Here's how the part is built. I have some questions about the finished solid (model axes, mm). Face numbers are marked on the shaded views. Coordinates: 2 decimals unless noted, no trailing zeros. Loops run counter-clockwise (first coordinate to the right, second up) from the corner with the lowest first, then second, coordinate; pieces in that order, holes last. Notation, with made-up numbers: (14, 0) -> (53, 0) arc R28 ccw to (53, 39) -> close; hole circle Ø8 at (43.25, 59). An arc over 180 degrees is marked (long way). Answer as a JSON object with one key per item and string values. Group by question number.
1) I'm going to push flat-ended pins straight in: pin 1 (5 mm diameter, centred on x = -3, z = 4, fed in from +Y); pin 2 (3 mm diameter, centred on x = -8.5, z = -15.5, fed in from -Y); pin 3 (3 mm diameter, centred on x = -3, y = 12, fed in from +Z). Where does each tip first touch, or does it pass through?
2) I want a section at C-C (y = 32.5). Write out the boundary of the cut face in (x, z) (3 decimals).
3) I want a section at B-B (z = 0). Count the separate pieces of the cut face and the enclosed holes in it, then the cut area to 3 significant figures.
4) I need wall thicknesses on probe 1 along Y at (x, z) = (-15.25, 0) (3 decimals); probe 2 along X at (y, z) = (12, 33); probe 3 along Y at (x, z) = (-4.75, 0). Which ranges of each line are inside material? Lowest first, please. Write a range as [from, to].
5) If we mould it in two halves opening along X, with no side actions, what happens to the marked faces 1, 2 and 3? For each: +X half, -X half, draft (parallel to the pull), parting line (faces both ways), or undercut.
6) I want a section at A-A (x = -2.5). Write out the boundary of the cut face in (y, z), then the cut area to 3 significant figures.
```python
from build123d import *

# Parameters (mm, degrees)
M2_5X0_45_TAPPED_HOLE2_D     = 2.05
M2_5X0_45_TAPPED_HOLE2_DEPTH = 6.35
M2_5X0_45_TAPPED_HOLE2_TIP   = 0.615882135
M3X0_5_TAPPED_HOLE1_D        = 2.5
M3X0_5_TAPPED_HOLE1_DEPTH    = 7.5
M3X0_5_TAPPED_HOLE1_TIP      = 0.751075774
CUT_EXTRUDE1_DEPTH           = 57.004464108


with BuildPart() as part:
    # Sketch1 → Revolve1 (revolve)
    with BuildSketch(Plane.XY, mode=Mode.PRIVATE) as revolve1_sk:
        Polygon((-18, 27.5), (0, 27.5), (0, 37.5), (-4, 37.5), (-4, 29.5), (-14, 29.5), (-14, 37.5), (-18, 37.5), align=None)
    revolve(revolve1_sk.sketch.rotate(Axis((0, 0, 0), (-1, 0, 0)), 90), axis=Axis((0, 0, 0), (-1, 0, 0)))

    # M2.5x0.45 Tapped Hole2
    with Locations(Plane.ZY.offset(18)):
        with Locations((0, -32.5), (-32.5, 0), (32.5, 0), (0, 32.5)):
            Hole(M2_5X0_45_TAPPED_HOLE2_D / 2, depth=M2_5X0_45_TAPPED_HOLE2_DEPTH)
            with Locations((0, 0, -(M2_5X0_45_TAPPED_HOLE2_DEPTH + M2_5X0_45_TAPPED_HOLE2_TIP / 2))):  # 118° drill point
                Cone(0, M2_5X0_45_TAPPED_HOLE2_D / 2, M2_5X0_45_TAPPED_HOLE2_TIP, mode=Mode.SUBTRACT)

    # M3x0.5 Tapped Hole1
    with Locations(Plane(origin=(0, 0, 0), x_dir=(0, 0, -1), z_dir=(1, 0, 0))):
        with Locations((-32.5, 0), (0, -32.5), (32.5, 0), (0, 32.5)):
            Hole(M3X0_5_TAPPED_HOLE1_D / 2, depth=M3X0_5_TAPPED_HOLE1_DEPTH)
            with Locations((0, 0, -(M3X0_5_TAPPED_HOLE1_DEPTH + M3X0_5_TAPPED_HOLE1_TIP / 2))):  # 118° drill point
                Cone(0, M3X0_5_TAPPED_HOLE1_D / 2, M3X0_5_TAPPED_HOLE1_TIP, mode=Mode.SUBTRACT)

    # Sketch8 → Cut-Extrude1 (cut, through all)
    with BuildSketch(Plane.ZY.offset(18)):
        Polygon((-27.223611076, 25.809397513), (-25.809397513, 27.223611076), (-18.725468962, 20.139682524), (-20.139682524, 18.725468962), align=None)
    extrude(amount=-CUT_EXTRUDE1_DEPTH, mode=Mode.SUBTRACT)


solid = part.part
```
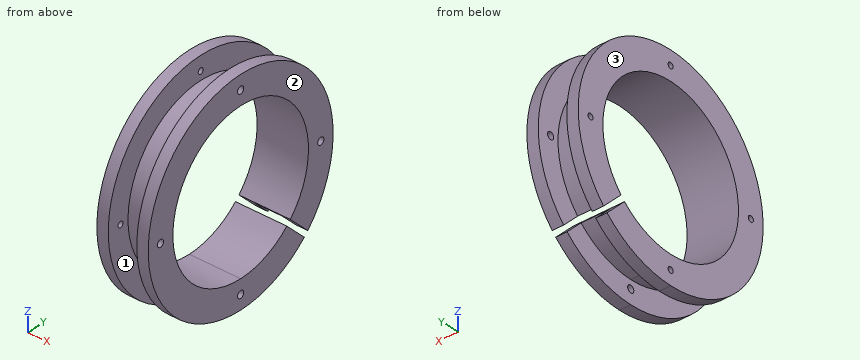
Determined:
{
 "1": {"pin 1": "y = 37.47", "pin 2": "y = -25.97", "pin 3": "z = 36"},
 "2": {"outline": "(-18, -18.708) -> (-14, -18.708) -> (-14, -1.025) -> (-18, -1.025) -> close; (-18, 1.025) -> (-14, 1.025) -> (-14, 18.708) -> (-18, 18.708) -> close; (-4, -18.708) -> (0, -18.708) -> (0, -1.25) -> (-4, -1.25) -> close; (-4, 1.25) -> (0, 1.25) -> (0, 18.708) -> (-4, 18.708) -> close"},
 "3": {"separate pieces": "6", "enclosed holes": "0", "area": "164 mm^2"},
 "4": {"probe 1": "[-37.5, -33.525], [-31.475, -27.5], [27.5, 31.475], [33.525, 37.5]", "probe 2": "[-18, -14], [-4, 0]", "probe 3": "[-29.5, -27.5], [27.5, 29.5]"},
 "5": {"face 1": "undercut", "face 2": "+X half", "face 3": "-X half"},
 "6": {"outline": "(18.73, -20.14) arc R27.5 cw (long way) to (20.14, -18.73) -> (27.21, -25.8) arc R37.5 ccw (long way) to (25.8, -27.21) -> close; hole circle Ø2.5 at (-32.5, 0); hole circle Ø2.5 at (0, -32.5); hole circle Ø2.5 at (0, 32.5); hole circle Ø2.5 at (32.5, 0)", "area": "2,000 mm^2"}
}
